Input: part model. Units: mm. Frame: model coordinates. Coordinates: 2 decimals unless noted, no trailing zeros. Loops run counter-clockwise (first coordinate to the right, second up) from the corner with the lowest first, then second, coordinate; pieces in that order, holes last. Notation, with made-up numbers: (30.5, 87.5) -> (85.5, 87.5) arc R11 cw to (85.5, 92.5) -> close; hole circle Ø8 at (28, -10.5). An arc over 180 degrees is marked (long way). Put each result on its own line as item: value. Start each with the question number.
1) Material intervals for L1, parallel to Z at x = -3.5, y = 31; L2, parallel to Z at x = 1.5, y = 47; L3, parallel to Y at x = -2.5, z = -17, sorted ascending.
2) Contact query for flat-ended pins moving along their axis: P1, Ø5, axis at x = 1, y = 38.5, coming from the -Z side; P2, Ø5, axis at x = -0.5, z = 30.5, coming from the +Y side; P3, Ø6, axis at x = -1.5, z = 12, coming from the +Y side; P4, Ø1.5, axis at y = 59.5, z = -51.5, coming from the -X side. Output: stop coordinate, or through.
3) Cut plane A-A (y = 37). Return the cut outline in (x, z).
4) Cut plane B-B (z = 0). Return the cut outline in (x, y).
from build123d import *

# Parameters (mm, degrees)
SKETCH_1_R                 = 24
EXTRUDE_1_DEPTH            = 5
SKETCH_2_R                 = 3
EXTRUDE_2_DEPTH            = 4
CHAMFER_1_SIZE             = 1
CHAMFER_1_OF_MIRROR_1_SIZE = 1
FILLET_1_R                 = 3


with BuildPart() as part:
    # 草圖1 → 伸長1 (new, symmetric)
    with BuildSketch(Plane(origin=(0, 0, 0), x_dir=(0, 0, -1), z_dir=(1, 0, 0))):
        with BuildLine():
            Line((-65, 45), (-65, 0))
            Line((-65, 0), (65, 0))
            Line((65, 0), (65, 45))
            ThreePointArc((65, 45), (0, 75), (-65, 45))
        make_face()
        with Locations((0, 37)):
            Circle(SKETCH_1_R, mode=Mode.SUBTRACT)
    extrude(amount=EXTRUDE_1_DEPTH, both=True)

    # 草圖2 → 伸長2 (add)
    with BuildSketch(Plane.XY.offset(65)):
        with Locations(Location((0, 32, 0), (0, 0, 180))):
            Circle(SKETCH_2_R)
        with Locations(Location((0, 17, 0), (0, 0, 180))):
            Circle(SKETCH_2_R)
    extrude_2 = extrude(amount=EXTRUDE_2_DEPTH)

    # 導角1
    chamfer_1_edges = [part.edges().sort_by_distance(p)[0] for p in [
        (3, 32, 69),
        (3, 17, 69),
    ]]
    chamfer(chamfer_1_edges, length=CHAMFER_1_SIZE)

    # 鏡射1: 伸長2 across plane
    add(extrude_2.mirror(Plane.XY))

    # 導角1 of 鏡射1
    chamfer_1_of_mirror_1_edges = [part.edges().sort_by_distance(p)[0] for p in [
        (3, 32, -69),
        (3, 17, -69),
    ]]
    chamfer(chamfer_1_of_mirror_1_edges, length=CHAMFER_1_OF_MIRROR_1_SIZE)

    # 圓角1
    fillet_1_edges = [part.edges().sort_by_distance(p)[0] for p in [
        (5, 0, 0),
        (-5, 37, 24),
        (5, 37, 24),
        (5, 75, 0),
        (-5, 0, 0),
        (-5, 75, 0),
    ]]
    fillet(fillet_1_edges, radius=FILLET_1_R)


solid = part.part
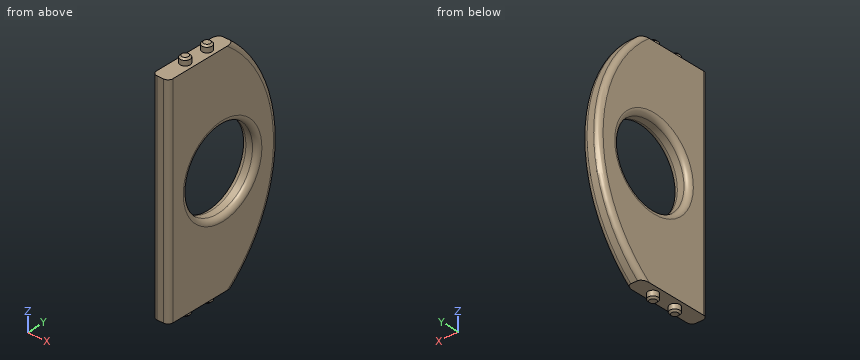
Results found:
1. L1: z = -65 to -23.65, 23.65 to 65
1. L2: z = -63.24 to -21.82, 21.82 to 63.24
1. L3: y = 0.04 to 20, 54 to 73.25
2. P1: stops at z = -65
2. P2: stops at y = 70.28
2. P3: stops at y = 74.52
2. P4: passes through
3. outline: (-5, -65) -> (5, -65) -> (5, -27) arc R3 ccw to (2, -24) -> (-2, -24) arc R3 ccw to (-5, -27) -> close; (-5, 27) arc R3 ccw to (-2, 24) -> (2, 24) arc R3 ccw to (5, 27) -> (5, 65) -> (-5, 65) -> close
4. outline: (-5, 3) arc R3 ccw to (-2, 0) -> (2, 0) arc R3 ccw to (5, 3) -> (5, 10) arc R3 ccw to (2, 13) -> (-2, 13) arc R3 ccw to (-5, 10) -> close; (-5, 64) arc R3 ccw to (-2, 61) -> (2, 61) arc R3 ccw to (5, 64) -> (5, 72) arc R3 ccw to (2, 75) -> (-2, 75) arc R3 ccw to (-5, 72) -> close
